from build123d import *

# Parameters (mm, degrees)
SKETCH_1_W          = 59
SKETCH_1_H          = 66
SKETCH_1_R          = 3.5
EXTRUDE_1_DEPTH     = 2.4
SKETCH_4_W          = 59
SKETCH_4_H          = 66
EXTRUDE_6_DEPTH     = 5.5
FILLET_1_R          = 5
FILLET_2_R          = 5
SKETCH_14_R         = 3
SKETCH_14_R_2       = 1.3
EXTRUDE_7_DEPTH     = 6.5
EXTRUDE_10_DEPTH    = 1
FILLET_3_R          = 1
CUT_EXTRUDE_1_DEPTH = 10
SKETCH_23_W         = 26.6
SKETCH_23_H         = 29.9
CUT_EXTRUDE_4_DEPTH = 52
SKETCH_24_W         = 26.6
SKETCH_24_H         = 5
EXTRUDE_11_DEPTH    = 0.2
SKETCH_25_W         = 26.6
SKETCH_25_H         = 5
EXTRUDE_12_DEPTH    = 0.2
SKETCH_26_R         = 3.14740537
SKETCH_26_R_2       = 1.3
EXTRUDE_13_DEPTH    = 6.5
SKETCH_27_R         = 4
CUT_EXTRUDE_5_DEPTH = 0.4
SKETCH_28_R         = 3.175170102
EXTRUDE_14_DEPTH    = 0.4
FILLET_4_R          = 0.5
FILLET_5_R          = 0.5


with BuildPart() as part:
    # Sketch 1 → Extrude 1 (new body)
    with BuildSketch(Plane.XY):
        with Locations((29.5, -33)):
            Rectangle(SKETCH_1_W, SKETCH_1_H)
        with Locations((12.36, -49.17)):
            Circle(SKETCH_1_R, mode=Mode.SUBTRACT)
    extrude(amount=EXTRUDE_1_DEPTH)

    # Sketch 4 → Extrude 6 (add)
    with BuildSketch(Plane.XY.offset(2.4)):
        with Locations((29.5, -33)):
            Rectangle(SKETCH_4_W, SKETCH_4_H)
        with BuildLine():
            Line((5.1, -2), (53.9, -2))
            ThreePointArc((53.9, -2), (56.092031022, -2.907968978), (57, -5.1))
            Line((57, -5.1), (57, -60.9))
            ThreePointArc((57, -60.9), (56.092031022, -63.092031022), (53.9, -64))
            Line((53.9, -64), (5.1, -64))
            ThreePointArc((5.1, -64), (2.907968978, -63.092031022), (2, -60.9))
            Line((2, -60.9), (2, -5.1))
            ThreePointArc((2, -5.1), (2.907968978, -2.907968978), (5.1, -2))
        make_face(mode=Mode.SUBTRACT)
    extrude(amount=EXTRUDE_6_DEPTH)

    # Fillet 1
    fillet_1_edges = [part.edges().sort_by_distance(p)[0] for p in [
        (0, 0, 3.95),
    ]]
    fillet(fillet_1_edges, radius=FILLET_1_R)

    # Fillet 2
    fillet_2_edges = [part.edges().sort_by_distance(p)[0] for p in [
        (59, 0, 3.95),
        (59, -66, 3.95),
        (0, -66, 3.95),
    ]]
    fillet(fillet_2_edges, radius=FILLET_2_R)

    # Sketch 14 → Extrude 7 (add)
    # profile 1 of 4: a face of its own
    with BuildSketch(Plane.XY.offset(2.4)):
        with Locations(Location((5, -5, 0), (0, 0, 180.947144451))):
            Circle(SKETCH_14_R)
        with Locations(Location((5, -5, 0), (0, 0, 180))):
            Circle(SKETCH_14_R_2, mode=Mode.SUBTRACT)
    # profile 2 of 4: a face of its own
    with BuildSketch(Plane.XY.offset(2.4)):
        with Locations(Location((5, -61, 0), (0, 0, 179.052855549))):
            Circle(SKETCH_14_R)
        with Locations(Location((5, -61, 0), (0, 0, 180))):
            Circle(SKETCH_14_R_2, mode=Mode.SUBTRACT)
    # profile 3 of 4: a face of its own
    with BuildSketch(Plane.XY.offset(2.4)):
        with Locations(Location((54, -61, 0), (0, 0, 269.052855549))):
            Circle(SKETCH_14_R)
        with Locations(Location((54, -61, 0), (0, 0, 180))):
            Circle(SKETCH_14_R_2, mode=Mode.SUBTRACT)
    # profile 4 of 4: a face of its own
    with BuildSketch(Plane.XY.offset(2.4)):
        with Locations(Location((54, -5, 0), (0, 0, 90.947144451))):
            Circle(SKETCH_14_R)
        with Locations(Location((54, -5, 0), (0, 0, 180))):
            Circle(SKETCH_14_R_2, mode=Mode.SUBTRACT)
    extrude(amount=EXTRUDE_7_DEPTH)

    # Fillet 3
    fillet_3_edges = [part.edges().sort_by_distance(p)[0] for p in [
        (0, -33, 0),
        (1.464466094, -1.464466094, 0),
        (29.5, -66, 0),
        (29.5, 0, 0),
        (59, -33, 0),
        (57.535533906, -1.464466094, 0),
        (57.535533906, -64.535533906, 0),
        (1.464466094, -64.535533906, 0),
    ]]
    fillet(fillet_3_edges, radius=FILLET_3_R)


with BuildPart() as body_2:
    # Sketch 15 → Extrude 10 (new body)
    with BuildSketch(Plane.XY.offset(7.9)):
        with BuildLine():
            Line((5, 0), (54, 0))
            ThreePointArc((54, 0), (57.535533906, -1.464466094), (59, -5))
            Line((59, -5), (59, -61))
            ThreePointArc((59, -61), (57.535533906, -64.535533906), (54, -66))
            Line((54, -66), (5, -66))
            ThreePointArc((5, -66), (1.464466094, -64.535533906), (0, -61))
            Line((0, -61), (0, -5))
            ThreePointArc((0, -5), (1.464466094, -1.464466094), (5, 0))
        make_face()
        with BuildLine():
            Line((5, -1), (54, -1))
            ThreePointArc((54, -1), (56.828427125, -2.171572875), (58, -5))
            Line((58, -5), (58, -61))
            ThreePointArc((58, -61), (56.828427125, -63.828427125), (54, -65))
            Line((54, -65), (5, -65))
            ThreePointArc((5, -65), (2.171572875, -63.828427125), (1, -61))
            Line((1, -61), (1, -5))
            ThreePointArc((1, -5), (2.171572875, -2.171572875), (5, -1))
        make_face(mode=Mode.SUBTRACT)
    extrude(amount=EXTRUDE_10_DEPTH)


with BuildPart() as cut_extrude_1_tool:
    # Sketch 20 → Cut-Extrude 1 (new body)
    with BuildSketch(Plane(origin=(59, 0, 0), x_dir=(0, 0, -1), z_dir=(1, 0, 0))):
        with BuildLine():
            Line((-8.9, -11.15), (-5.2, -11.15))
            ThreePointArc((-5.2, -11.15), (-4.492893219, -11.442893219), (-4.2, -12.15))
            Line((-4.2, -12.15), (-4.2, -18.25))
            ThreePointArc((-4.2, -18.25), (-4.492893219, -18.957106781), (-5.2, -19.25))
            Line((-5.2, -19.25), (-8.9, -19.25))
            Line((-8.9, -19.25), (-8.9, -11.15))
        make_face()
    extrude(amount=-CUT_EXTRUDE_1_DEPTH)


with BuildPart() as part_1:
    add(part.part)

    # Cut-Extrude 1: cut by cut_extrude_1_tool
    add(cut_extrude_1_tool.part, mode=Mode.SUBTRACT)

    # Sketch 23 → Cut-Extrude 4 (cut)
    with BuildSketch(Plane(origin=(0, 0, 0), x_dir=(-1, 0, 0), z_dir=(0, 0, -1))):
        with Locations((-29.500023272, -22.190991649)):
            Rectangle(SKETCH_23_W, SKETCH_23_H)
    extrude(amount=-CUT_EXTRUDE_4_DEPTH, mode=Mode.SUBTRACT)

    # Sketch 24 → Extrude 11 (add)
    with BuildSketch(Plane.XY.offset(2.4)):
        with Locations((29.500023272, -4.740991649)):
            Rectangle(SKETCH_24_W, SKETCH_24_H)
    extrude(amount=EXTRUDE_11_DEPTH)

    # Sketch 25 → Extrude 12 (add)
    with BuildSketch(Plane.XY.offset(2.4)):
        with Locations((29.500023272, -39.640991649)):
            Rectangle(SKETCH_25_W, SKETCH_25_H)
    extrude(amount=EXTRUDE_12_DEPTH)


with BuildPart() as body_2_1:
    add(body_2.part)

    # Cut-Extrude 1: cut by cut_extrude_1_tool
    add(cut_extrude_1_tool.part, mode=Mode.SUBTRACT)


    add(part_1.part)  # Extrude 13 merges part
    # Sketch 26 → Extrude 13 (add)
    with BuildSketch(Plane.XY.offset(2.4)):
        with Locations(Location((46.9, -5.7, 0), (0, 0, 180))):
            Circle(SKETCH_26_R)
        with Locations(Location((46.9, -5.7, 0), (0, 0, 180))):
            Circle(SKETCH_26_R_2, mode=Mode.SUBTRACT)
    extrude(amount=EXTRUDE_13_DEPTH)

    # Sketch 27 → Cut-Extrude 5 (cut)
    with BuildSketch(Plane(origin=(0, 0, 0), x_dir=(-1, 0, 0), z_dir=(0, 0, -1))):
        with Locations((-44.3, -54.4)):
            Circle(SKETCH_27_R)
    extrude(amount=-CUT_EXTRUDE_5_DEPTH, mode=Mode.SUBTRACT)

    # Sketch 28 → Extrude 14 (add)
    with BuildSketch(Plane(origin=(0, 0, 0.4), x_dir=(-1, 0, 0), z_dir=(0, 0, -1))):
        with Locations((-44.3, -54.4)):
            Circle(SKETCH_28_R)
    extrude(amount=EXTRUDE_14_DEPTH)

    # Fillet 4
    # the kernel refuses this fillet: 0.5 mm, written as the material it takes off along each edge
    with BuildSketch(Plane(origin=(44.3, -54.4, 0), x_dir=(-1, 0, 0), z_dir=(0, -1, 0))) as fillet_4_piece_1:
        with BuildLine():
            CenterArc((4.489897949, -0.5), FILLET_4_R, 90, 78.463040967)
            Line((4, -0.4), (3.990202041, -0.398))
            ThreePointArc((3.990202041, -0.398), (3.99, -0.2), (3.99, 0))
            Line((3.99, 0), (4, 0.01))
            Line((4, 0.01), (4.489897949, 0.01))
            Line((4.489897949, 0.01), (4.489897949, 0))
        make_face()
    revolve(axis=Axis((44.3, -54.4, 0), (0, 0, -1)), mode=Mode.SUBTRACT)

    # Fillet 5
    # the kernel refuses this fillet: 0.5 mm, written as the material it takes off along each edge
    with BuildSketch(Plane(origin=(44.3, -54.4, 0), x_dir=(-1, 0, 0), z_dir=(0, -1, 0))) as fillet_5_piece_1:
        with BuildLine():
            CenterArc((2.685272154, -0.5), FILLET_5_R, 11.536959033, 78.463040967)
            Line((2.685272154, 0), (2.685272154, 0.01))
            Line((2.685272154, 0.01), (3.175170102, 0.01))
            Line((3.175170102, 0.01), (3.185170102, 0))
            ThreePointArc((3.185170102, 0), (3.185170102, -0.2), (3.184968061, -0.398))
            Line((3.184968061, -0.398), (3.175170102, -0.4))
        make_face()
    revolve(axis=Axis((44.3, -54.4, 0), (0, 0, -1)), mode=Mode.SUBTRACT)


solid = body_2_1.part
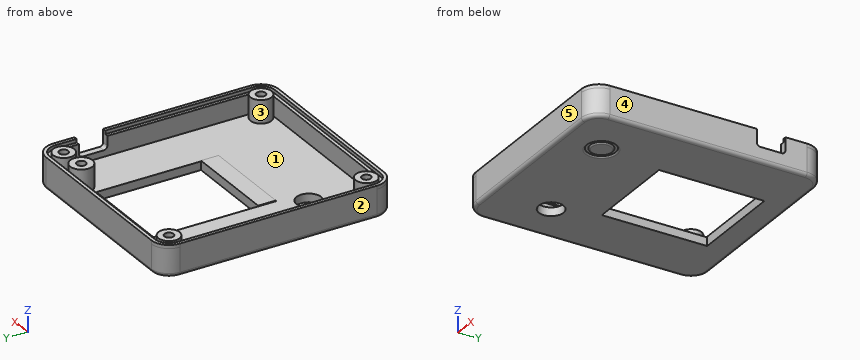
Can you work these out from the model? Positions are in its coordinate system, mm. Face numbers are marked on the shaded views. A direction names the side the tool comes from. Round coordinates to 2 decimals unless told otherwise and drop trailing zeros. Write each loop counter-clockwise with the first axis right and the second up, starting at its lowest first coordinate (ties: lowest second). Pieces come first, ordered by that corner, then holes. Notation, with made-up numbers: (-7.5, 15.5) -> (14.5, 15.5) arc R18 cw to (14.5, 38.5) -> close; hole circle Ø5 at (25, 64). An arc over 180 degrees is marked (long way). Use one line per item in the form item = value. Start each with the question number.
Q1. I'm going to push flat-ended pins straight in: P1, Ø1.6, axis at x = 5, y = -61, coming from the +Z side; P2, Ø2.5, axis at x = 28, y = -40, coming from the +Z side; P3, Ø17, axis at x = 30, y = -20.5, coming from the +Z side; P4, Ø2, axis at x = 58.5, y = -14, coming from the +Z side. Where does each tip first touch, or does it pass through?
Q2. Imagine slicing it at A-A (z = 7). Count the separate pieces of the cut face and the enclosed holes in it, then the cut area to 3 significant figures.
Q3. Imagine slicing it at C-C (y = -49.17). Please give me the cut outline in (x, z), then the cut area to 3 significant figures.
Q4. We'd pull the mould along X, two halves only. Please class the marked faces 3, 4 and 5: +X half, -X half, draft (parallel to the pull), parting line (faces both ways), or undercut.
Q5. Which directions (+Z, -Z, +X, -X, +Y, -Y) give clear straight access to the entire face, cutting with the end or side of a thin tool? Please do the marked faces 1 and 2.
Q6. Imagine slicing it at B-B (x = 12.36). Please give me the cut outline in (y, z).
Q7. If I drill on probe 1 along Y at (x, z) = (54, 4); probe 2 along Y at (x, z) = (46.9, 6.25); probe 3 along X at (y, z) = (-61, 4.25), over which ranges is the centre line in solid material (lowest first)? Write a range as [from, to].
Q8. Imagine slicing it at D-D (x = 23). Please give me the cut outline in (y, z), then the cut area to 3 significant figures.
Worked out:
q1.P1 = 2.4
q1.P2 = 2.6
q1.P3 = through
q1.P4 = 4.2
q2.separate_pieces = 2
q2.enclosed_holes = 5
q2.area = 572 mm^2
q3.outline = (0, 1) arc R1 ccw to (1, 0) -> (8.86, 0) -> (8.86, 2.4) -> (2, 2.4) -> (2, 7.9) -> (1, 7.9) -> (1, 8.9) -> (0, 8.9) -> close; (15.86, 0) -> (58, 0) arc R1 ccw to (59, 1) -> (59, 8.9) -> (58, 8.9) -> (58, 7.9) -> (57, 7.9) -> (57, 2.4) -> (15.86, 2.4) -> close
q3.area = 148 mm^2
q4.face_3 = undercut
q4.face_4 = +X half
q4.face_5 = draft
q5.face_1 = +Z
q5.face_2 = +Z, -Z, -X, +Y, -Y
q6.outline = (-66, 1) arc R1 ccw to (-65, 0) -> (-52.67, 0) -> (-52.67, 2.4) -> (-64, 2.4) -> (-64, 7.9) -> (-65, 7.9) -> (-65, 8.9) -> (-66, 8.9) -> close; (-45.67, 0) -> (-1, 0) arc R1 ccw to (0, 1) -> (0, 8.9) -> (-1, 8.9) -> (-1, 7.9) -> (-2, 7.9) -> (-2, 2.4) -> (-45.67, 2.4) -> close
q7.probe_1 = [-66, -62.3], [-59.7, -58], [-8, -6.3], [-3.7, 0]
q7.probe_2 = [-66, -64], [-8.85, -7], [-4.4, -2.55], [-2, 0]
q7.probe_3 = [0, 3.7], [6.3, 8], [51, 52.7], [55.3, 59]
q8.outline = (-66, 1) arc R1 ccw to (-65, 0) -> (-37.14, 0) -> (-37.14, 2.6) -> (-42.14, 2.6) -> (-42.14, 2.4) -> (-64, 2.4) -> (-64, 7.9) -> (-65, 7.9) -> (-65, 8.9) -> (-66, 8.9) -> close; (-7.24, 0) -> (-1, 0) arc R1 ccw to (0, 1) -> (0, 8.9) -> (-1, 8.9) -> (-1, 7.9) -> (-2, 7.9) -> (-2, 2.4) -> (-2.24, 2.4) -> (-2.24, 2.6) -> (-7.24, 2.6) -> close
q8.area = 112 mm^2
